CAD build for the part. Positions are in the model's coordinates, mm. A direction names the side the tool comes from. Coordinates: 2 decimals unless noted, no trailing zeros. Loops run counter-clockwise (first coordinate to the right, second up) from the corner with the lowest first, then second, coordinate; pieces in that order, holes last. Notation, with made-up numbers: (20.25, 39.5) -> (38.25, 39.5) arc R15 ccw to (38.25, 57.5) -> close; hole circle Ø3 at (87.5, 12.5). An arc over 180 degrees is marked (long way). Answer as CSV lines item,"result". Start each with the question number.
```python
from build123d import *

# Parameters (mm, degrees)
BOSS_EXTRUDE1_DEPTH = 10
SKETCH2_R           = 1.25
BOSS_EXTRUDE2_DEPTH = 5
SKETCH3_R           = 1.25
BOSS_EXTRUDE3_DEPTH = 5


with BuildPart() as part:
    # Sketch1 → Boss-Extrude1 (new body)
    with BuildSketch(Plane.XY):
        with BuildLine():
            Line((0, 0), (80, 0))
            ThreePointArc((80, 0), (90, -10), (80, -20))
            Line((80, -20), (25, -20))
            ThreePointArc((25, -20), (15, -30), (25, -40))
            Line((25, -40), (80, -40))
            ThreePointArc((80, -40), (90, -50), (80, -60))
            Line((80, -60), (0, -60))
            Line((0, -60), (0, -55))
            Line((0, -55), (80, -55))
            ThreePointArc((80, -55), (85, -50), (80, -45))
            Line((80, -45), (25, -45))
            ThreePointArc((25, -45), (10, -30), (25, -15))
            Line((25, -15), (80, -15))
            ThreePointArc((80, -15), (85, -10), (80, -5))
            Line((80, -5), (0, -5))
            Line((0, -5), (0, 0))
        make_face()
    extrude(amount=BOSS_EXTRUDE1_DEPTH)

    # Sketch2 → Boss-Extrude2 (add)
    with BuildSketch(Plane.ZY):
        with Locations(Location((5, -2.5, 0), (0, 0, 180))):
            Circle(SKETCH2_R)
    extrude(amount=BOSS_EXTRUDE2_DEPTH)

    # Sketch3 → Boss-Extrude3 (add)
    with BuildSketch(Plane.ZY):
        with Locations(Location((5, -57.5, 0), (0, 0, 180))):
            Circle(SKETCH3_R)
    extrude(amount=BOSS_EXTRUDE3_DEPTH)


solid = part.part
```
Q1. Saw through at A-A (x = 50.5). List the corners of the cut face in (y, z).
Q2. Saw through at B-B (z = 8.25). List the corners of the cut face in (x, y), and give its area (3 significant figures).
Q3. Which spindle directions (+Z, -Z, +X, -X, +Y, -Y) get a long thin tool onto all of the face, cutting with end or side? Do faces 5 (the flat face through (53, -20, 5)), 6 (the cylindrical face through (-2.46, -58.74, 5.16)), 7 (the flat face through (53, -45, 5)). Say none if no direction does.
Q4. Pin check, flat tips, straight feed: pin 1 Ø3 at (x, z) = (51.5, 3.5) entering from +Y; pin 2 Ø6 at (y, z) = (-30.5, 6) entering from -X; pin 3 Ø3 at (x, y) = (20.5, -23) entering from +Z; pin 4 Ø5 at (y, z) = (-9, 4.5) entering from -X. Stop position of each tip, or through.
Q5. Probe probe 1 along Y at (x, z) = (31, 6.75); probe 2 along Y at (x, z) = (84, 8.25); probe 3 along Y at (x, z) = (9.5, 5.5). List the from-to ranges inside material, lowest first. Write a range as from..to.
Q6. Two-plate mould, pull along Y, no slides. Class faces 1 (the flat face through (39, 0, 5)), 2 (the flat face through (-5, -58, 5)), 3 (the cylindrical face through (85, -50, 5)), 4 (the cylindrical face through (90, -10, 5)): pulls with the +Y half, pulls with the -Y half, needs draft (parallel to the pull), parting line crosses it, or undercut.
Q7. Saw through at C-C (x = 8.5). List the corners of the cut face in (y, z), and give its area (3 significant figures).
Q8. Saw through at D-D (y = -2.5). List the corners of the cut face in (x, z).
Ans:
1,outline,"(-60, 0) -> (-55, 0) -> (-55, 10) -> (-60, 10) -> close; (-45, 0) -> (-40, 0) -> (-40, 10) -> (-45, 10) -> close; (-20, 0) -> (-15, 0) -> (-15, 10) -> (-20, 10) -> close; (-5, 0) -> (0, 0) -> (0, 10) -> (-5, 10) -> close"
2,outline,"(0, -60) -> (80, -60) arc R10 ccw to (80, -40) -> (25, -40) arc R10 cw to (25, -20) -> (80, -20) arc R10 ccw to (80, 0) -> (0, 0) -> (0, -5) -> (80, -5) arc R5 cw to (80, -15) -> (25, -15) arc R15 ccw to (25, -45) -> (80, -45) arc R5 cw to (80, -55) -> (0, -55) -> close"
2,area,"1,780 mm²"
3,face 5,"+Z, -Z, +X"
3,face 6,"-X"
3,face 7,"+Z, -Z, -X"
4,pin 1,"stops at y = 0"
4,pin 2,"stops at x = 10"
4,pin 3,"passes through"
4,pin 4,"stops at x = 83.57"
5,probe 1,"y = -60..-55, -45..-40, -20..-15, -5..0"
5,probe 2,"y = -59.17..-53, -47..-40.83, -19.17..-13, -7..-0.83"
5,probe 3,"y = -60..-55, -5..0"
6,face 1,"pulls with the +Y half"
6,face 2,"needs draft"
6,face 3,"undercut"
6,face 4,"undercut"
7,outline,"(-60, 0) -> (-55, 0) -> (-55, 10) -> (-60, 10) -> close; (-5, 0) -> (0, 0) -> (0, 10) -> (-5, 10) -> close"
7,area,"100 mm²"
8,outline,"(-5, 3.75) -> (0, 3.75) -> (0, 0) -> (86.61, 0) -> (86.61, 10) -> (0, 10) -> (0, 6.25) -> (-5, 6.25) -> close"
